from build123d import *

# Parameters (mm, degrees)
SKIZZE1_W                            = 57
SKIZZE1_H                            = 123
AUFSATZ_LINEAR_AUSTRAGEN1_DEPTH      = 2.5
SCHNITT_LINEAR_AUSTRAGEN1_DEPTH      = 84.889808678
SCHNITT_LINEAR_AUSTRAGEN2_DEPTH      = 68.828828679
SCHNITT_LINEAR_AUSTRAGEN3_DEPTH      = 70.726045338
SCHNITT_LINEAR_AUSTRAGEN3_DEPTH_BACK = 70.726045338
SCHNITT_LINEAR_AUSTRAGEN4_DEPTH      = 70.47454308
SCHNITT_LINEAR_AUSTRAGEN4_DEPTH_BACK = 70.47454308
SCHNITT_LINEAR_AUSTRAGEN5_DEPTH      = 68.828828679


with BuildPart() as part:
    # Skizze1 → Aufsatz-Linear austragen1 (new body)
    with BuildSketch(Plane(origin=(0, 0, 0), x_dir=(1, 0, 0), z_dir=(0, 1, 0))):
        Rectangle(SKIZZE1_W, SKIZZE1_H)
    extrude(amount=AUFSATZ_LINEAR_AUSTRAGEN1_DEPTH)

    # Skizze2 → Schnitt-Linear austragen1 (cut, through all)
    with BuildSketch(Plane(origin=(28.5, 0, 0), x_dir=(0, 0, -1), z_dir=(1, 0, 0))):
        Polygon((-61.5, 2.5), (-61.5, 0), (-60.968608596, 0), align=None)
    extrude(amount=-SCHNITT_LINEAR_AUSTRAGEN1_DEPTH, mode=Mode.SUBTRACT)

    # Skizze3 → Schnitt-Linear austragen2 (cut, through all)
    with BuildSketch(Plane(origin=(0, 2.5, 0), x_dir=(1, 0, 0), z_dir=(0, 1, 0))):
        Polygon((-28.5, -61.5), (-17.738894386, 61.5), (-28.5, 61.5), align=None)
        Polygon((28.5, -61.5), (17.738894386, 61.5), (28.5, 61.5), align=None)
    extrude(amount=-SCHNITT_LINEAR_AUSTRAGEN2_DEPTH, mode=Mode.SUBTRACT)

    # Skizze5 → Schnitt-Linear austragen3 (cut, two sides: drawn at the far end of the back side and taken through both)
    with BuildSketch(Plane(origin=(0.175618176, 0, 2.007324937), x_dir=(0, -1, 0), z_dir=(0.08715574274765484, 0, 0.9961946980917459)).offset(-SCHNITT_LINEAR_AUSTRAGEN3_DEPTH_BACK)):
        Polygon((0.008562414, 23.031470717), (-2.5, 23.031470717), (0, 21.995936811), align=None)
    extrude(amount=SCHNITT_LINEAR_AUSTRAGEN3_DEPTH + SCHNITT_LINEAR_AUSTRAGEN3_DEPTH_BACK, mode=Mode.SUBTRACT)

    # Skizze6 → Schnitt-Linear austragen4 (cut, two sides: drawn at the far end of the back side and taken through both)
    with BuildSketch(Plane(origin=(-0.152372814, 0, 1.741629235), x_dir=(0, 1, 0), z_dir=(-0.08715574274766175, 0, 0.9961946980917452)).offset(-SCHNITT_LINEAR_AUSTRAGEN4_DEPTH_BACK)):
        Polygon((2.5, 23.031470717), (0, 21.995936811), (0, 23.031470717), align=None)
    extrude(amount=SCHNITT_LINEAR_AUSTRAGEN4_DEPTH + SCHNITT_LINEAR_AUSTRAGEN4_DEPTH_BACK, mode=Mode.SUBTRACT)

    # Skizze8 → Schnitt-Linear austragen5 (cut, through all)
    with BuildSketch(Plane(origin=(0, 2.5, 0), x_dir=(1, 0, 0), z_dir=(0, 1, 0))):
        with BuildLine():
            Line((17.738894386, 61.5), (9.738894386, 61.5))
            Line((9.738894386, 61.5), (9.738894386, 44.5))
            Line((9.738894386, 44.5), (9.738894386, 44.494341137))
            ThreePointArc((9.738894386, 44.494341137), (12.660237078, 37.430870976), (19.717416528, 34.494364202))
            Line((19.717416528, 34.494364202), (20.101653571, 34.493538941))
            Line((20.101653571, 34.493538941), (17.738894386, 61.5))
        make_face()
    extrude(amount=-SCHNITT_LINEAR_AUSTRAGEN5_DEPTH, mode=Mode.SUBTRACT)


solid = part.part
Source: CAD feature listing. Evaluate the final solid. Frame: model axes, mm. A direction names the side the tool comes from. Coordinates: 2 decimals unless noted, no trailing zeros. Loops run counter-clockwise (first coordinate to the right, second up) from the corner with the lowest first, then second, coordinate; pieces in that order, holes last. Notation, with made-up numbers: (55.5, 54) - (114.5, 54) arc R11 cw to (114.5, 60) - close; hole circle Ø2 at (32.25, -11.75). An arc over 180 degrees is marked (long way). Return JSON: item names as keys, results as strings.
Q1. Access query for faces 1 (the flat face through (0.4, 1.23, 61.23)), 2 (the flat face through (9.739, 1, -53)). Directions: +Z, -Z, +X, -X, +Y, -Y. A direction counts if a zero-diameter tool reaches every point of the face in a straight line with its end or side. Return the directions, or none.
Results:
{"face 1": "+Z, +X, -X, -Y", "face 2": "-Z, +X, +Y, -Y"}
Q2. Section A-A, the plane y = 0.4. Return loops of the section in (x, z).
Results:
{"outline": "(-27.59, 61.05) - (-16.87, -61.5) - (9.74, -61.5) - (9.74, -44.49) arc R10 cw to (19.23, -34.51) - (27.59, 61.05) - close"}
Q3. Section C-C, the plane x = -24.5. Return loops of the section in (y, z).
Results:
{"outline": "(0, 27.66) - (2.5, 15.78) - (2.5, 61.5) - (0, 60.97) - close"}
Q4. Material intervals for line 1 along Y through (x, z) = (26.5, 43); line 2 along X through (y, z) = (2.1, -12.5); line 3 along Z through (x, y) = (-14.5, 1.2), sorted ascending.
Results:
{"line 1": "1.58 to 2.5", "line 2": "-21.86 to 21.86", "line 3": "-61.5 to 61.22"}
Q5. Contact query for flat-ended pins moving along their axis: P1, Ø1, axis at x = -7, y = 0.5, coming from the +Z side; P2, Ø1, axis at y = 1.5, z = 43, coming from the +X side. Output: stop coordinate, or through.
Results:
{"P1": "z = 61.18", "P2": "x = 26.68"}
Q6. Section B-B, the plane z = 8. Return loops of the section in (x, y).
Results:
{"outline": "(-23.82, 2.5) - (-22.78, 0) - (22.78, 0) - (23.82, 2.5) - close"}
